Could you check a few things on this drawing? It's one solid part, dimensions in mm from its lowest x, y, z. Round coordinates to 2 decimals unless told otherwise and drop trailing zeros. Loops run counter-clockwise (first coordinate to the right, second up) from the corner with the lowest first, then second, coordinate; pieces in that order, holes last. Notation, with made-up numbers: M 52.5,79 L 60.5,79 A26 ccw 60.5,95 Z; hole C -26,1 d8. An arc over 180 degrees is marked long. Put each result on its own line as item: value. Start each with the question number.
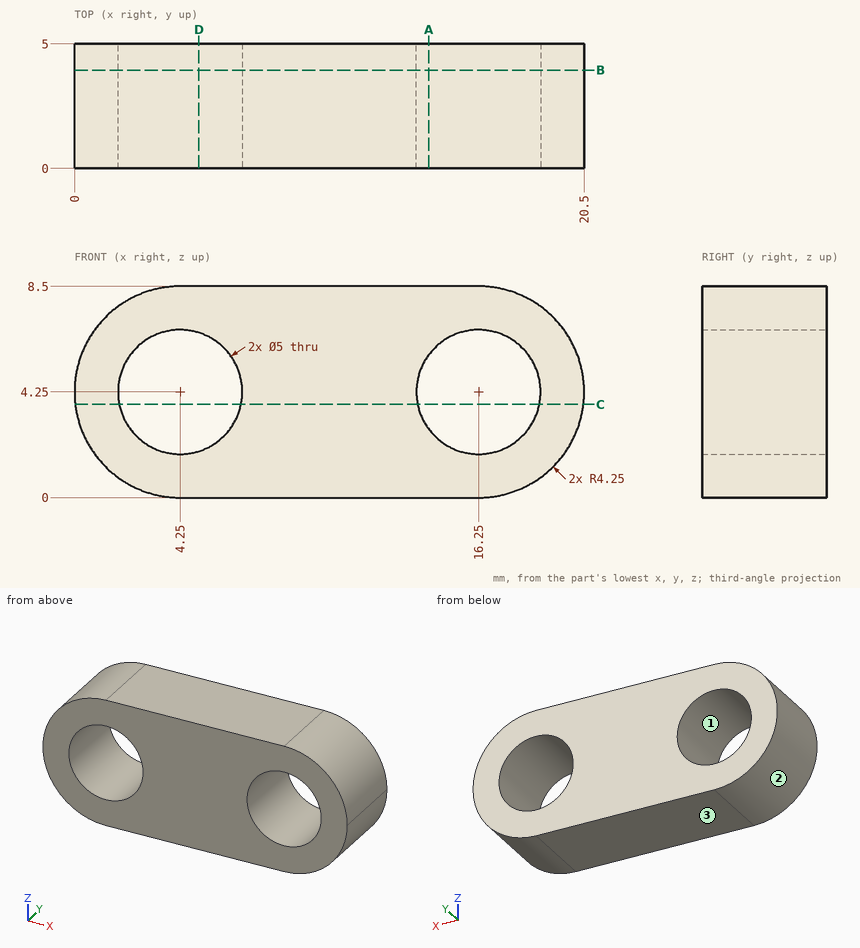
1) If we mould it in two halves opening along X, with no side actions, what happens to the marked faces 1, 2 and 3? For each: pulls with the +X half, pulls with the -X half, needs draft (parallel to the pull), parting line crosses it, or undercut.
2) Suppose I cut it at C-C (z = 3.75). Write out the boundary of the cut face in (x, y).
3) Suppose I cut it at D-D (x = 5). Write out the boundary of the cut face in (y, z), plus the area to 3 significant figures.
4) If I drill on probe 1 along X at (y, z) = (3.95, 3.5); probe 2 along X at (y, z) = (1.15, 3); probe 3 along Z at (x, y) = (4.5, 3.4), over which ranges is the centre line in solid material (lowest first)? Write a range as from..to.
5) Suppose I cut it at B-B (y = 3.95). Write out the boundary of the cut face in (x, z).
6) Suppose I cut it at A-A (x = 14.25). Write out the boundary of the cut face in (y, z).
7) I'm going to push flat-ended pins straight in: P1, Ø1.5, axis at y = 1.5, z = 5.5, coming from the -X side; P2, Ø3, axis at x = 4.25, z = 4.25, coming from the +Y side; P3, Ø1, axis at y = 1, z = 1.5, coming from the +X side. Where does each tip first touch, or does it pass through?
Results are:
1. face 1: undercut
1. face 2: pulls with the -X half
1. face 3: needs draft
2. outline: M 0.03,0 L 1.8,0 L 1.8,5 L 0.03,5 Z; M 6.7,0 L 13.8,0 L 13.8,5 L 6.7,5 Z; M 18.7,0 L 20.47,0 L 20.47,5 L 18.7,5 Z
3. outline: M 0,0 L 5,0 L 5,1.87 L 0,1.87 Z; M 0,6.63 L 5,6.63 L 5,8.5 L 0,8.5 Z
3. area: 18.7 mm²
4. probe 1: 0.07..1.87, 6.63..13.87, 18.63..20.43
4. probe 2: 0.19..2.08, 6.42..14.08, 18.42..20.31
4. probe 3: 0..1.76, 6.74..8.5
5. outline: M 4.25,0 L 16.25,0 A4.25 ccw 20.5,4.25 A4.25 ccw 16.25,8.5 L 4.25,8.5 A4.25 ccw Z; hole C 4.25,4.25 d5; hole C 16.25,4.25 d5
6. outline: M 0,0 L 5,0 L 5,2.75 L 0,2.75 Z; M 0,5.75 L 5,5.75 L 5,8.5 L 0,8.5 Z
7. P1: x = 0.03
7. P2: through
7. P3: x = 19.86
